```python
from build123d import *

# Parameters (mm, degrees)
F2_R     = 1.5
F3_DEPTH = 25
F4_SIZE  = 0.5


with BuildPart() as f1:
    # F0 (on Front) → F1 (revolve)
    with BuildSketch(Plane.XZ):
        Polygon((0, 130), (0, 0), (3.5, 0), (3.5, 10), (5, 10), (5, 13), (4.5, 13), (4.5, 14), (5, 14), (5, 17), (4.5, 17), (4.5, 18), (5, 18), (5, 21), (4.5, 21), (4.5, 22), (5, 22), (5, 25), (4.5, 25), (4.5, 98), (5, 98), (5, 101), (4.5, 101), (4.5, 102), (5, 102), (5, 105), (4.5, 105), (4.5, 106), (5, 106), (5, 109), (4.5, 109), (4.5, 110), (5, 110), (5, 113), (4.5, 113), (4.5, 114), (5, 114), (5, 115), (2.5, 130), align=None)
    revolve(axis=Axis((0, 0, 65), (0, 0, 1)))

    # F2 (on face) → F3 (cut)
    with BuildSketch(Plane.XY.offset(130)):
        Circle(F2_R)
    extrude(amount=-F3_DEPTH, mode=Mode.SUBTRACT)

    # F4
    f4_edges = [f1.edges().sort_by_distance(p)[0] for p in [
        (-3.5, 0, 0),
    ]]
    chamfer(f4_edges, length=F4_SIZE)


solid = f1.part
```
Geometry: final body of the model. Coordinates: model frame, mm. A direction names the side the tool comes from. Round coordinates to 2 decimals unless told otherwise and drop trailing zeros. Loops run counter-clockwise (first coordinate to the right, second up) from the corner with the lowest first, then second, coordinate; pieces in that order, holes last. Notation, with made-up numbers: (74.25, 8) -> (89.25, 8) arc R16 ccw to (89.25, 29) -> close; hole circle Ø7 at (75.5, 75). An arc over 180 degrees is marked (long way). Use one line per item in the form item = value.
Item 1: Material intervals for probe 1 along Y at (x, z) = (0, 114.25); probe 2 along Y at (x, z) = (0, 116.25); probe 3 along Z at (x, y) = (0, 1.25), sorted ascending.
Evaluation:
probe_1 = -5 to -1.5, 1.5 to 5
probe_2 = -4.79 to -1.5, 1.5 to 4.79
probe_3 = 0 to 105
Item 2: Contact query for flat-ended pins moving along their axis: pin 1 Ø3 at (y, z) = (0.5, 83.5) entering from +X; pin 2 Ø2.5 at (x, y) = (0, 0) entering from +Z; pin 3 Ø6 at (x, z) = (-3, 36.5) entering from -Y. Output: stop coordinate, or through.
Evaluation:
pin_1 = 4.5
pin_2 = 105
pin_3 = -4.5
Item 3: Cut plane A-A on z = 57. Output: boundary loops of the cut face in (x, y), then the cut area to 3 significant figures.
Evaluation:
outline = circle Ø9 at (0, 0)
area = 63.6 mm2
Item 4: Draft query along Y for faces 1 (the flat face through (-2.2, -3.3, 10)), 2 (the cylindrical face through (-1.08, -4.88, 19.52)), 3 (the cylindrical face through (-1.5, 0.07, 117.68)). Return one class per face: released by +Y, released by -Y, zero draft, split by the parting line, or undercut.
Evaluation:
face_1 = zero draft
face_2 = split by the parting line
face_3 = undercut
Item 5: Access query for faces 4 (the cylindrical face through (-1.08, -4.88, 111.52)), 5 (the cylindrical face through (-0.59, 4.46, 17.51)), 6 (the cylindrical face through (3.233, -1.341, 5.316)). Directions: +Z, -Z, +X, -X, +Y, -Y. A direction counts if a zero-diameter tool reaches every point of the face in a straight line with its end or side. Return the directions, or none.
Evaluation:
face_4 = +Z, -Z
face_5 = none
face_6 = -Z
